from build123d import *

# Parameters (mm, degrees)
F0_R     = 51.918659
F1_DEPTH = 8
F2_DEPTH = 20


with BuildPart() as f1:
    # F0 (on Top) → F1 (new body)
    with BuildSketch(Plane.XY):
        Circle(F0_R)
        with BuildLine():
            ThreePointArc((10.300017, 14.557494), (15.838083, 8.195493), (17.832863, 0))
            ThreePointArc((17.832863, 0), (15.838083, -8.195493), (10.300017, -14.557494))
            ThreePointArc((10.300017, -14.557494), (0, -17.832863), (-10.300017, -14.557494))
            ThreePointArc((-10.300017, -14.557494), (-17.832863, 0), (-10.300017, 14.557494))
            ThreePointArc((-10.300017, 14.557494), (0, 17.832863), (10.300017, 14.557494))
        make_face(mode=Mode.SUBTRACT)
        with BuildLine():
            Line((-10.300017, -14.557494), (-10.300017, 14.557494))
            ThreePointArc((-10.300017, 14.557494), (-17.832863, 0), (-10.300017, -14.557494))
        make_face()
        with BuildLine():
            ThreePointArc((10.300017, -14.557494), (15.838083, -8.195493), (17.832863, 0))
            ThreePointArc((17.832863, 0), (15.838083, 8.195493), (10.300017, 14.557494))
            Line((10.300017, 14.557494), (10.300017, -14.557494))
        make_face()
    extrude(amount=F1_DEPTH)

    # F0 (on Top) → F2 (join)
    with BuildSketch(Plane.XY):
        with BuildLine():
            Line((-10.300017, -14.557494), (-10.300017, 14.557494))
            ThreePointArc((-10.300017, 14.557494), (-17.832863, 0), (-10.300017, -14.557494))
        make_face()
        with BuildLine():
            ThreePointArc((10.300017, -14.557494), (15.838083, -8.195493), (17.832863, 0))
            ThreePointArc((17.832863, 0), (15.838083, 8.195493), (10.300017, 14.557494))
            Line((10.300017, 14.557494), (10.300017, -14.557494))
        make_face()
    extrude(amount=F2_DEPTH)


solid = f1.part
Read the model definition and answer for the solid it produces. Units are mm, in the model's axes. A direction names the side the tool comes from. Give positions to 0.01 mm unless a question says otherwise; leave off trailing zeros. Write each loop counter-clockwise with the first axis right and the second up, starting at its lowest first coordinate (ties: lowest second). Pieces come first, ordered by that corner, then holes. Notation, with made-up numbers: (-5, 9) - (52, 9) arc R20 ccw to (52, 47) - close; hole circle Ø6 at (10.25, 47.25). An arc over 180 degrees is marked (long way). Answer in a Markdown table with one row per item. Add a question column.
Item 1: Section B-B, the plane x = 0 is taken. Write down the section's boundary in (y, z), and give its area (3 significant figures).
Item 2: Find the intervals of material crossed by L1, parallel to X at y = -0.5, z = 18.5; L2, parallel to Z at x = -10, y = 29; L3, parallel to Y at x = 3, z = 7.25, in increasing order.
Item 3: Section C-C, the plane y = 7.5 is taken. Write down the section's boundary in (x, z), and give its area (3 significant figures).
Item 4: A tool of negligible diameter and unlimited length cuts with its end or side. For faces 4 (the face through (11, 1, 0)), 5 (the face through (-0.154, 17.832, 3.944)), from which of +Z, -Z, +X, -X, +Y, -Y can it reach the whole face along a straight path? Write none if from no direction.
Item 5: Flat-ended cylindrical pins translate along their axes: P1, Ø4, axis at y = 1, z = 5, coming from the -X side; P2, Ø12, axis at y = 6.5, z = 17, coming from the -X side; P3, Ø12, axis at x = 31, z = 10.5, coming from the +Y side; P4, Ø10, axis at x = -38.5, y = -11, coming from the +Z side. Find the tip coordinate at first contact, or state that the pin passes through.
Item 6: Section A-A, the plane z = 12.75 is taken. Write down the section's boundary in (x, y), and give its area (3 significant figures).
Item 7: Section D-D, the plane z = 6.5 is taken. Write down the section's boundary in (x, y), and give its area (3 significant figures).
Item 8: Determine the mould class of faces 1 (the face through (13, 0, 20)), 2 (the face through (-10.3, 0, 10)), 3 (the face through (-17.83, 0.24, 13.92)) for opening direction Y: pulls with the +Y half, pulls with the -Y half, needs draft (parallel to the pull), parting line crosses it, or undercut.
Recorded:
| question | item | result |
|---|---|---|
| 1 | outline | (-51.92, 0) - (-17.83, 0) - (-17.83, 8) - (-51.92, 8) - close; (17.83, 0) - (51.92, 0) - (51.92, 8) - (17.83, 8) - close |
| 1 | area | 545 mm2 |
| 2 | L1 | x = -17.83 to -10.3, 10.3 to 17.83 |
| 2 | L2 | z = 0 to 8 |
| 2 | L3 | y = -51.83 to -17.58, 17.58 to 51.83 |
| 3 | outline | (-51.37, 0) - (-10.3, 0) - (-10.3, 20) - (-16.18, 20) - (-16.18, 8) - (-51.37, 8) - close; (10.3, 0) - (51.37, 0) - (51.37, 8) - (16.18, 8) - (16.18, 20) - (10.3, 20) - close |
| 3 | area | 798 mm2 |
| 4 | face 4 | -Z, +X, -X, +Y, -Y |
| 4 | face 5 | +Z, -Z |
| 5 | P1 | stops at x = -51.92 |
| 5 | P2 | stops at x = -17.83 |
| 5 | P3 | stops at y = 45.2 |
| 5 | P4 | stops at z = 8 |
| 6 | outline | (-10.3, -14.56) - (-10.3, 14.56) arc R17.83 ccw to start; (10.3, -14.56) arc R17.83 ccw to (17.83, 0) arc R17.83 ccw to (10.3, 14.56) - close |
| 6 | area | 308 mm2 |
| 7 | outline | circle Ø103.84 at (0, 0); hole (-10.3, -14.56) arc R17.83 ccw to (10.3, -14.56) - (10.3, 14.56) arc R17.83 ccw to (-10.3, 14.56) - close |
| 7 | area | 7,780 mm2 |
| 8 | face 1 | needs draft |
| 8 | face 2 | undercut |
| 8 | face 3 | parting line crosses it |
